from build123d import *

# Parameters (mm, degrees)
EXTRUDE_1_DEPTH     = 5
CUT_EXTRUDE_1_DEPTH = 6
FILLET_1_R          = 2
FILLET_2_R          = 2
FILLET_3_R          = 3
FILLET_4_R          = 3
FILLET_5_R          = 3
FILLET_6_R          = 2
FILLET_7_R          = 1
FILLET_8_R          = 1
FILLET_9_R          = 1
FILLET_10_R         = 1
FILLET_11_R         = 2
FILLET_12_R         = 2
FILLET_13_R         = 2
FILLET_14_R         = 2
FILLET_15_R         = 2
FILLET_16_R         = 2


with BuildPart() as part:
    # 草图1 → 凸台-拉伸1 (new body)
    with BuildSketch(Plane(origin=(0, 0, 0), x_dir=(1, 0, 0), z_dir=(0, 1, 0))):
        Polygon((-5, 5), (0, 5), (0, 0), (10, 0), (10, 5), (40, 5), (40, 0), (50, 0), (50, 5), (55, 5), (55, 10), (39, 10), (33.75, 85.078497848), (16.25, 85.078497848), (12.482276941, 31.197547838), (-1.715229851, 31.197547838), (-35.526844906, 50.718692892), (-40.526844906, 42.058438854), (15, 10), (-5, 10), align=None)
    extrude(amount=EXTRUDE_1_DEPTH)

    # 草图2 → 切除-拉伸1 (cut, through all)
    with BuildSketch(Plane(origin=(0, 5, 0), x_dir=(1, 0, 0), z_dir=(0, 1, 0))):
        Polygon((-35.854277493, 42.247482146), (-27.194023456, 37.247482146), (-24.694023456, 41.577609165), (-33.354277493, 46.577609165), align=None)
        Polygon((28.868403571, 71.682200114), (23.868403571, 80.342454152), (19.538276552, 77.842454152), (24.538276552, 69.182200114), align=None)
        Polygon((-3.054975814, 26.197547838), (17, 26.197547838), (17, 14.618802154), align=None)
        Polygon((20.75, 63.374046916), (29.25, 63.374046916), (31.5, 31.197547838), (18.5, 31.197547838), align=None)
        Polygon((22, 26.197547838), (22, 10), (32.855147628, 26.197547838), align=None)
    extrude(amount=-CUT_EXTRUDE_1_DEPTH, mode=Mode.SUBTRACT)

    # 圆角1
    fillet_1_edges = [part.edges().sort_by_distance(p)[0] for p in [
        (20.75, 2.5, -63.374046916),
    ]]
    fillet(fillet_1_edges, radius=FILLET_1_R)

    # 圆角2
    fillet_2_edges = [part.edges().sort_by_distance(p)[0] for p in [
        (29.25, 2.5, -63.374046916),
    ]]
    fillet(fillet_2_edges, radius=FILLET_2_R)

    # 圆角3
    fillet_3_edges = [part.edges().sort_by_distance(p)[0] for p in [
        (18.5, 2.5, -31.197547838),
    ]]
    fillet(fillet_3_edges, radius=FILLET_3_R)

    # 圆角4
    fillet_4_edges = [part.edges().sort_by_distance(p)[0] for p in [
        (31.5, 2.5, -31.197547838),
    ]]
    fillet(fillet_4_edges, radius=FILLET_4_R)

    # 圆角5
    fillet_5_edges = [part.edges().sort_by_distance(p)[0] for p in [
        (22, 2.5, -26.197547838),
    ]]
    fillet(fillet_5_edges, radius=FILLET_5_R)

    # 圆角6
    fillet_6_edges = [part.edges().sort_by_distance(p)[0] for p in [
        (32.855147628, 2.5, -26.197547838),
    ]]
    fillet(fillet_6_edges, radius=FILLET_6_R)

    # 圆角7
    fillet_7_edges = [part.edges().sort_by_distance(p)[0] for p in [
        (22, 2.5, -10),
    ]]
    fillet(fillet_7_edges, radius=FILLET_7_R)

    # 圆角8
    fillet_8_edges = [part.edges().sort_by_distance(p)[0] for p in [
        (17, 2.5, -14.618802154),
    ]]
    fillet(fillet_8_edges, radius=FILLET_8_R)

    # 圆角9
    fillet_9_edges = [part.edges().sort_by_distance(p)[0] for p in [
        (-3.054975814, 2.5, -26.197547838),
    ]]
    fillet(fillet_9_edges, radius=FILLET_9_R)

    # 圆角10
    fillet_10_edges = [part.edges().sort_by_distance(p)[0] for p in [
        (17, 2.5, -26.197547838),
    ]]
    fillet(fillet_10_edges, radius=FILLET_10_R)

    # 圆角11
    fillet_11_edges = [part.edges().sort_by_distance(p)[0] for p in [
        (-5, 2.5, -10),
    ]]
    fillet(fillet_11_edges, radius=FILLET_11_R)

    # 圆角12
    fillet_12_edges = [part.edges().sort_by_distance(p)[0] for p in [
        (55, 2.5, -10),
    ]]
    fillet(fillet_12_edges, radius=FILLET_12_R)

    # 圆角13
    fillet_13_edges = [part.edges().sort_by_distance(p)[0] for p in [
        (39, 2.5, -10),
    ]]
    fillet(fillet_13_edges, radius=FILLET_13_R)

    # 圆角14
    fillet_14_edges = [part.edges().sort_by_distance(p)[0] for p in [
        (15, 2.5, -10),
    ]]
    fillet(fillet_14_edges, radius=FILLET_14_R)

    # 圆角15
    fillet_15_edges = [part.edges().sort_by_distance(p)[0] for p in [
        (-40.526844906, 2.5, -42.058438854),
        (-35.526844906, 2.5, -50.718692892),
    ]]
    fillet(fillet_15_edges, radius=FILLET_15_R)

    # 圆角16
    fillet_16_edges = [part.edges().sort_by_distance(p)[0] for p in [
        (33.75, 2.5, -85.078497848),
        (-1.715229851, 2.5, -31.197547838),
        (12.482276941, 2.5, -31.197547838),
        (16.25, 2.5, -85.078497848),
    ]]
    fillet(fillet_16_edges, radius=FILLET_16_R)


solid = part.part
Source: CAD feature listing. Evaluate the final solid. Frame: model axes, mm. A direction names the side the tool comes from. Coordinates: 2 decimals unless noted, no trailing zeros. Write each loop counter-clockwise with the first axis right and the second up, starting at its lowest first coordinate (ties: lowest second). Pieces come first, ordered by that corner, then holes. Notation, with made-up numbers: M -20.75,24.25 L -5.75,24.25 A33 ccw -5.75,58.25 Z; hole C 62,39 d8. An arc over 180 degrees is marked long. Use a Markdown table: item, result.
1) Ray query, L1, parallel to Z at x = 26.5, y = 1.7; L2, parallel to X at y = 3.4, z = -44; L3, parallel to Z at x = 23, y = 2.25. Return the intervals inside material, ascending.
Conclusion:
| item | result |
|---|---|
| L1 | z = -85.08 to -75.78, -70.31 to -63.37, -31.2 to -26.2, -16.71 to -5 |
| L2 | x = -39.41 to -34.84, -28.89 to -23.89, 13.38 to 19.4, 30.6 to 36.62 |
| L3 | z = -85.08 to -79.84, -71.85 to -63.37, -31.2 to -25.43, -12.29 to -5 |
2) Reachability of faces 5 (the flat face through (-3, 2, -5)), 6 (the flat face through (50, 2, -2)), 7 (the cylindrical face through (21.236, 2.465, -62.822)) from +Z, -Z, +X, -X, +Y, -Y: full face, straight path, thin tool, end or side. Return the list, or none.
Conclusion:
| item | result |
|---|---|
| face 5 | +Z, -X, +Y, -Y |
| face 6 | +Z, +X, +Y, -Y |
| face 7 | +Y, -Y |
3) Section C-C, the plane y = 4. Give the number of separate pieces and of enclosed holes in the cut face, then the cut area to 3 significant figures.
Conclusion:
| item | result |
|---|---|
| separate pieces | 1 |
| enclosed holes | 5 |
| area | 2,100 mm^2 |
4) First-contact query: pin 1 Ø2.5 at (y, z) = (2.5, -3.5) entering from +X; pin 2 Ø3 at (y, z) = (2, -29) entering from +X; pin 3 Ø1 at (y, z) = (4, -44.5) entering from +X; pin 4 Ø5 at (x, z) = (41.5, -41.5) entering from -Y. Flat tips, straight axial feed; report the tip coordinate or a pass-through.
Conclusion:
| item | result |
|---|---|
| pin 1 | stops at x = 50 |
| pin 2 | stops at x = 37.78 |
| pin 3 | stops at x = 36.62 |
| pin 4 | passes through |
5) Section A-A, the plane z = -51.5. Output: boundary loops of the cut face in (x, y), then the cut area to 3 significant figures.
Conclusion:
| item | result |
|---|---|
| outline | M 13.9,0 L 19.92,0 L 19.92,5 L 13.9,5 Z; M 30.08,0 L 36.1,0 L 36.1,5 L 30.08,5 Z |
| area | 60.2 mm^2 |
6) Section B-B, the plane x = 46. Output: boundary loops of the cut face in (y, z), then the cut area to 3 significant figures.
Conclusion:
| item | result |
|---|---|
| outline | M 0,-10 L 5,-10 L 5,0 L 0,0 Z |
| area | 50.0 mm^2 |
7) Mould query, pull axis X, two halves, no side actions, for faces 1 (the flat face through (2, 2, -10)), 2 (the flat face through (14.39, 2.46, -58.49)), 3 (the cylindrical face through (33.23, 2.54, -84.56)), 4 (the flat face through (0, 2, -3)). Classes: pulls with the +X half, pulls with the -X half, needs draft (parallel to the pull), parting line crosses it, or undercut.
Conclusion:
| item | result |
|---|---|
| face 1 | needs draft |
| face 2 | undercut |
| face 3 | pulls with the +X half |
| face 4 | pulls with the -X half |
8) Section D-D, the plane x = -20. Output: boundary loops of the cut face in (y, z).
Conclusion:
| item | result |
|---|---|
| outline | M 0,-41.75 L 5,-41.75 L 5,-30.21 L 0,-30.21 Z |
